Check sheet for the drawn part. Datum: minimum x, y, z corner. Units: mm. Coordinates: 2 decimals unless noted, no trailing zeros. Loops run counter-clockwise (first coordinate to the right, second up) from the corner with the lowest first, then second, coordinate; pieces in that order, holes last. Notation, with made-up numbers: (-40, 64.25) - (-14, 64.25) arc R13 cw to (-14, 85.25) - close; hole circle Ø9 at (75.25, 17.5). An arc over 180 degrees is marked (long way). Answer as CSV lines item,"result". Start each with the question number.
1. Cross-section at A-A (x = 25). Enter the section's corners in (y, z).
2. Cross-section at D-D (x = 15). Enter the section's corners in (y, z).
3. Cross-section at B-B (y = 1.5). Enter the section's corners in (x, z).
4. Material ranges on line 1 (X direction, y = 0.95, z = 22.85); line 2 (X direction, y = 1.3, z = 47.5); line 3 (X direction, y = 0.3, z = 45.5), recorded low to high. Write a range as [from, to].
5. Cross-section at C-C (z = 46). Enter the section's corners in (x, y), plus the area to 3 significant figures.
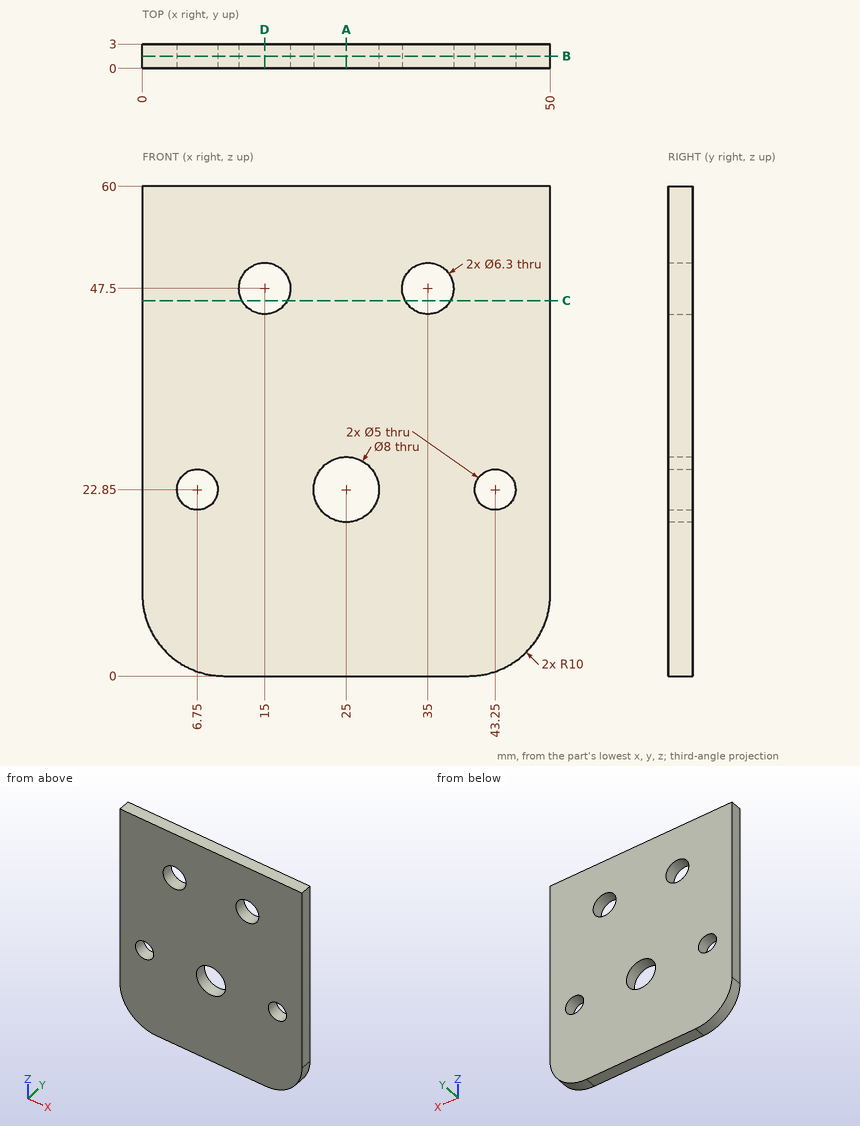
Values follow:
1,outline,"(0, 0) - (3, 0) - (3, 18.85) - (0, 18.85) - close; (0, 26.85) - (3, 26.85) - (3, 60) - (0, 60) - close"
2,outline,"(0, 0) - (3, 0) - (3, 44.35) - (0, 44.35) - close; (0, 50.65) - (3, 50.65) - (3, 60) - (0, 60) - close"
3,outline,"(0, 10) arc R10 ccw to (10, 0) - (40, 0) arc R10 ccw to (50, 10) - (50, 60) - (0, 60) - close; hole circle Ø5 at (6.75, 22.85); hole circle Ø6.3 at (15, 47.5); hole circle Ø8 at (25, 22.85); hole circle Ø6.3 at (35, 47.5); hole circle Ø5 at (43.25, 22.85)"
4,line 1,"x = [0, 4.25], [9.25, 21], [29, 40.75], [45.75, 50]"
4,line 2,"x = [0, 11.85], [18.15, 31.85], [38.15, 50]"
4,line 3,"x = [0, 12.57], [17.43, 32.57], [37.43, 50]"
5,outline,"(0, 0) - (12.23, 0) - (12.23, 3) - (0, 3) - close; (17.77, 0) - (32.23, 0) - (32.23, 3) - (17.77, 3) - close; (37.77, 0) - (50, 0) - (50, 3) - (37.77, 3) - close"
5,area,"117 mm²"
